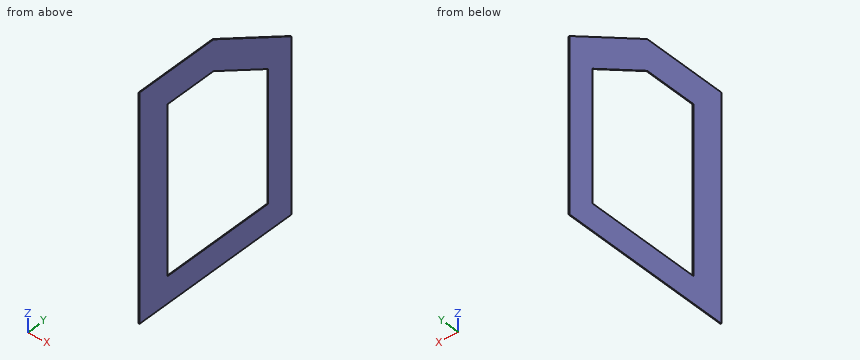
```python
from build123d import *

# Parameters (mm, degrees)
BOSS_EXTRUDE1_DEPTH = 3.175
CUT_EXTRUDE1_REACH  = 5.175


with BuildPart() as part:
    # Sketch1 → Boss-Extrude1 (new body)
    with BuildSketch(Plane(origin=(0, 0, 0), x_dir=(0, 0, -1), z_dir=(1, 0, 0))):
        Polygon((0, 0), (-822.266180236, 0), (-1066.8, -423.545), (-1066.8, -826.77), (0, -826.77), align=None)
    extrude(amount=BOSS_EXTRUDE1_DEPTH)

    # Sketch2 → Cut-Extrude1 (cut, up to next)
    with BuildSketch(Plane(origin=(3.175, 0, 0), x_dir=(0, 0, -1), z_dir=(1, 0, 0)), mode=Mode.PRIVATE) as cut_extrude1_sk1:
        Polygon((-748.942696049, -127), (-920.153031626, -423.545), (-920.153031626, -674.37), (-127, -674.37), (-127, -423.545), (-127, -127), align=None)
    cut_extrude1_tool1 = extrude(cut_extrude1_sk1.sketch, amount=-CUT_EXTRUDE1_REACH, mode=Mode.PRIVATE) & part.part
    add(cut_extrude1_tool1.solids().sort_by_distance((3.175, -411.543058, 502.491806))[0], mode=Mode.SUBTRACT)


solid = part.part
```
Design review of the part built by this model. Coordinates are the model's own, in mm. Round coordinates to 2 decimals unless told otherwise and drop trailing zeros. Write each loop counter-clockwise with the first axis right and the second up, starting at its lowest first coordinate (ties: lowest second). Pieces come first, ordered by that corner, then holes. Notation, with made-up numbers: (65.25, 48.25) -> (115.25, 48.25) arc R19 cw to (115.25, 85.25) -> close; hole circle Ø9 at (47, 87). An arc over 180 degrees is marked (long way). Write item = value, one per line. Start each with the question number.
1) Take a section at A-A, the plane z = 228. State the section outline as (x, y) points (3 decimals).
2) Take a section at C-C, the plane y = -165.5. State the section outline as (x, z) points (3 decimals).
3) Clearance check with flat-ended pins moving along their axes: pin 1 (1 mm diameter, centred on x = 2.5, y = -297.5, fed in from +Z); pin 2 (1 mm diameter, centred on x = 1, y = -353, fed in from -Z). State where each tip first meets the part, or that it passes through.
4) Wall thickness on probe 1 along Z at (x, y) = (0.95, -508); probe 2 along Y at (x, z) = (1.8, 676); probe 3 along Z at (x, y) = (1.8, -347): over which ranges is each line inside the solid? List them lowest first. Write a range as from..to.
5) Take a section at B-B, the plane x = 1.1. State the section outline as (y, z) points (3 decimals).
Results list:
q1.outline = (0, -826.77) -> (3.175, -826.77) -> (3.175, -674.37) -> (0, -674.37) -> close; (0, -127) -> (3.175, -127) -> (3.175, 0) -> (0, 0) -> close
q2.outline = (0, 0) -> (3.175, 0) -> (3.175, 127) -> (0, 127) -> close; (0, 771.171) -> (3.175, 771.171) -> (3.175, 917.818) -> (0, 917.818) -> close
q3.pin_1 = 994.32
q3.pin_2 = 0
q4.probe_1 = 0..127, 920.15..1066.8
q4.probe_2 = -826.77..-674.37, -127..0
q4.probe_3 = 0..127, 875.96..1022.61
q5.outline = (-826.77, 0) -> (0, 0) -> (0, 822.266) -> (-423.545, 1066.8) -> (-826.77, 1066.8) -> close; hole (-674.37, 127) -> (-127, 127) -> (-127, 748.943) -> (-423.545, 920.153) -> (-674.37, 920.153) -> close
